Geometry: final body of the model. Coordinates: model frame, mm. A direction names the side the tool comes from. Give positions to 0.01 mm unless a question says otherwise; leave off trailing zeros. Write each loop counter-clockwise with the first axis right and the second up, starting at its lowest first coordinate (ties: lowest second). Pieces come first, ordered by that corner, then holes. Notation, with made-up numbers: (-26.5, 60.5) -> (-17.5, 60.5) arc R16 cw to (-17.5, 87.5) -> close; hole circle Ø8 at (-33.5, 66). An arc over 180 degrees is marked (long way). Use CSV: the item, a comma, the result in double quotes. Start each with the question number.
1) Section A-A (z = 43). Output: boundary loops of the cut face in (x, y), plus the area to 3 significant figures.
2) Material intervals for line 1 (Z direction, x = -0.75, y = 8); line 2 (Y direction, x = -0.5, z = 59); line 3 (Z direction, x = -2.25, y = -1), sorted ascending. Write a range as [from, to].
3) Set-up query: faces 1 (the face through (0, 0, 69)), 2 (the face through (4, 0, 68.2)). Return all of +Z, -Z, +X, -X, +Y, -Y with unobstructed straight access to the full face (end or side cutting, diameter ignored); none if empty.
4) Contact query for flat-ended pins moving along their axis: P1, Ø1, axis at x = -4.5, y = 1.5, coming from the +Z side; P2, Ø1.5, axis at x = 2, z = 53, coming from the -Y side; P3, Ø1.5, axis at x = 3, z = 24, coming from the -Y side. Output: stop coordinate, or through.
```python
from build123d import *

# Parameters (mm, degrees)
F0_R     = 9.15
F0_R_2   = 3.1
F1_DEPTH = 68.2
F2_DEPTH = 69


# Not quite as in the source:
# - a fillet or chamfer that OpenCascade refuses, or shapes differently, is made with other operations: its cross-section is extruded or revolved along the edge and cut away or added


with BuildPart() as f1:
    # F0 (on Top) → F1 (new body)
    with BuildSketch(Plane.XY):
        Circle(F0_R)
        Circle(F0_R_2, mode=Mode.SUBTRACT)
    extrude(amount=F1_DEPTH)

    # F0 (on Top) → F2 (join)
    with BuildSketch(Plane.XY):
        Circle(F0_R_2)
    extrude(amount=F2_DEPTH)

    # F3: fillet of radius 1 on 3 edges, made by hand

    # F3_s1 → F3_t2 (revolve, cut)
    with BuildSketch(Plane.XZ):
        with BuildLine():
            ThreePointArc((3.1, 68.2), (2.7526596349, 68.7745966692), (2.1202041029, 69))
            Line((2.1202041029, 69), (3.1, 69))
            Line((3.1, 69), (3.1, 68.2))
        make_face()
    revolve(axis=Axis((0, 0, 69), (0, 0, 1)), mode=Mode.SUBTRACT)

    # F3_s3 → F3_t4 (revolve, cut)
    with BuildSketch(Plane.XZ):
        with BuildLine():
            ThreePointArc((9.15, 67.2), (8.8571067812, 67.9071067812), (8.15, 68.2))
            Line((8.15, 68.2), (9.15, 68.2))
            Line((9.15, 68.2), (9.15, 67.2))
        make_face()
    revolve(axis=Axis((0, 0, 68.2), (0, 0, 1)), mode=Mode.SUBTRACT)

    # F3_s5 → F3_t6 (revolve, cut)
    with BuildSketch(Plane.XZ):
        with BuildLine():
            ThreePointArc((9.15, 1), (8.8571067812, 0.2928932188), (8.15, 0))
            Line((8.15, 0), (9.15, 0))
            Line((9.15, 0), (9.15, 1))
        make_face()
    revolve(axis=Axis((0, 0, 0), (0, 0, 1)), mode=Mode.SUBTRACT)


solid = f1.part
```
Answers follow:
1,outline,"circle Ø18.3 at (0, 0)"
1,area,"263 mm^2"
2,line 1,"z = [0, 68.2]"
2,line 2,"y = [-9.14, 9.14]"
2,line 3,"z = [0, 68.94]"
3,face 1,"+Z, +X, -X, +Y, -Y"
3,face 2,"+Z"
4,P1,"stops at z = 68.2"
4,P2,"stops at y = -9.06"
4,P3,"stops at y = -8.87"
